The listing builds one solid part. Answer for the finished solid, in the listing's coordinates (mm). Coordinates: 2 decimals unless noted, no trailing zeros. Order: outer loops, then holes, each group sorted by start corner. A loop starts at its lowest first (then second) coordinate and runs counter-clockwise, first axis right, second up.
from build123d import *

# Parameters (mm, degrees)
SKETCH1_W           = 80
SKETCH1_H           = 80
BOSS_EXTRUDE1_DEPTH = 7
SKETCH2_R           = 2.5
CUT_EXTRUDE1_DEPTH  = 10
SKETCH4_W           = 80
SKETCH4_H           = 7
BOSS_EXTRUDE2_DEPTH = 35
SKETCH3_R           = 1.5
SKETCH3_R_2         = 12.5
CUT_EXTRUDE2_DEPTH  = 10


with BuildPart() as part:
    # Sketch1 → Boss-Extrude1 (new body)
    with BuildSketch(Plane(origin=(0, 0, 0), x_dir=(1, 0, 0), z_dir=(0, 1, 0))):
        with Locations((40, 40)):
            Rectangle(SKETCH1_W, SKETCH1_H)
    extrude(amount=BOSS_EXTRUDE1_DEPTH)

    # Sketch2 → Cut-Extrude1 (cut)
    with BuildSketch(Plane.XZ):
        with Locations(Location((70, -70, 0), (0, 0, 270))):
            Circle(SKETCH2_R)
        with Locations(Location((70, -10, 0), (0, 0, 270))):
            Circle(SKETCH2_R)
        with Locations(Location((10, -10, 0), (0, 0, 270))):
            Circle(SKETCH2_R)
        with Locations(Location((10, -70, 0), (0, 0, 270))):
            Circle(SKETCH2_R)
    extrude(amount=-CUT_EXTRUDE1_DEPTH, mode=Mode.SUBTRACT)

    # Sketch4 → Boss-Extrude2 (add)
    with BuildSketch(Plane(origin=(80, 0, 0), x_dir=(0, 0, -1), z_dir=(1, 0, 0))):
        with Locations((40, 3.5)):
            Rectangle(SKETCH4_W, SKETCH4_H)
    extrude(amount=BOSS_EXTRUDE2_DEPTH)

    # Sketch3 → Cut-Extrude2 (cut)
    with BuildSketch(Plane.XZ):
        with Locations(Location((107.5, -24.5, 0), (0, 0, 270))):
            Circle(SKETCH3_R)
        with Locations(Location((107.5, -55.5, 0), (0, 0, 270))):
            Circle(SKETCH3_R)
        with Locations(Location((76.5, -55.5, 0), (0, 0, 270))):
            Circle(SKETCH3_R)
        with Locations(Location((76.5, -24.5, 0), (0, 0, 270))):
            Circle(SKETCH3_R)
        with Locations(Location((92, -40, 0), (0, 0, 270))):
            Circle(SKETCH3_R_2)
    extrude(amount=-CUT_EXTRUDE2_DEPTH, mode=Mode.SUBTRACT)


solid = part.part
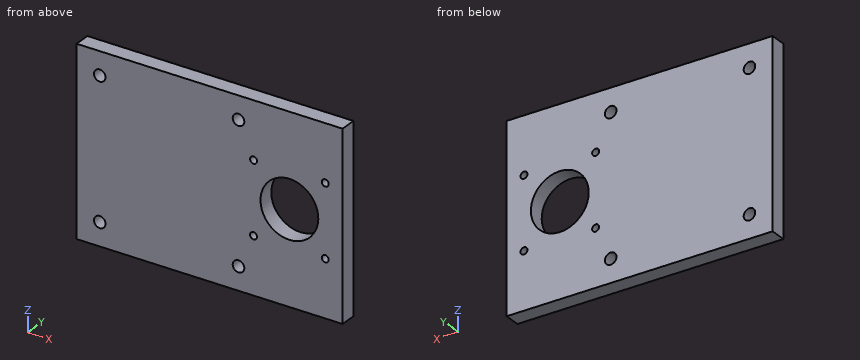
(1) Find section C-C on z = -55.5. Determine the outline of the cut face in (x, y).
(2) Given pin 1 Ø1.8 at (x, z) = (76.5, -55.5) entering from -Y, flat-ended and moving along its own axis, determine where the tip first touches the part or whether it passes through.
(3) Find the intervals of material crossed by probe 1 along X at (y, z) = (2, -55.5); probe 2 along X at (y, z) = (2, -70); probe 3 along Z at (x, y) = (11, 6.75), in increasing order.
(4) Find section A-A on z = -40. Determine the outline of the cut face in (x, y).
(5) Find section D-D on y = 1.75. Count the separate pieces of the cut face and the enclosed holes in it, then the cut area to 3 significant figures.
(6) Find section B-B on x = 99.5. Determine the outline of the cut face in (y, z).
Resolved:
1. outline: (0, 0) - (75, 0) - (75, 7) - (0, 7) - close; (78, 0) - (106, 0) - (106, 7) - (78, 7) - close; (109, 0) - (115, 0) - (115, 7) - (109, 7) - close
2. pin 1: passes through
3. probe 1: x = 0 to 75, 78 to 106, 109 to 115
3. probe 2: x = 0 to 7.5, 12.5 to 67.5, 72.5 to 115
3. probe 3: z = -80 to -72.29, -67.71 to -12.29, -7.71 to 0
4. outline: (0, 0) - (79.5, 0) - (79.5, 7) - (0, 7) - close; (104.5, 0) - (115, 0) - (115, 7) - (104.5, 7) - close
5. separate pieces: 1
5. enclosed holes: 9
5. area: 8,600 mm2
6. outline: (0, -80) - (7, -80) - (7, -50) - (0, -50) - close; (0, -30) - (7, -30) - (7, 0) - (0, 0) - close
